from build123d import *

# Parameters (mm, degrees)
F0_W     = 31
F0_H     = 70
F0_H_2   = 17
F0_H_3   = 50
F0_H_4   = 20
F1_DEPTH = 0.4


with BuildPart() as f1:
    # F0 (on Top) → F1 (new body, symmetric)
    with BuildSketch(Plane.XY):
        Polygon((-8.5, -35), (8.5, -35), (13.5, 15), (8.5, 35), (-8.5, 35), align=None)
        with Locations((-24, 0)):
            Rectangle(F0_W, F0_H)
        with Locations((-24, -43.5)):
            Rectangle(F0_W, F0_H_2)
        Polygon((-56.5, -35), (-39.5, -35), (-39.5, 35), (-56.5, 35), (-61.5, 15), align=None)
        with Locations((-24, -77)):
            Rectangle(F0_W, F0_H_3)
        with Locations((-24, -112)):
            Rectangle(F0_W, F0_H_4)
        with Locations((-24, -130.5)):
            Rectangle(F0_W, F0_H_2)
    extrude(amount=F1_DEPTH, both=True)


solid = f1.part
Can you work these out from the model? Positions are in its coordinate system, mm. Round coordinates to 2 decimals unless told otherwise and drop trailing zeros. Loops run counter-clockwise (first coordinate to the right, second up) from the corner with the lowest first, then second, coordinate; pieces in that order, holes last. Notation, with made-up numbers: (88, -8.5) - (143, -8.5) arc R8 ccw to (143, -4.5) - close; hole circle Ø7 at (-29.5, 89.5). An arc over 180 degrees is marked (long way). Answer in a Markdown table with one row per item. Add a question column.
Q1. I want a section at A-A on z = 0.15. List the corners of the cut face in (x, y) for me.
Q2. I want a section at C-C on y = -7.5. List the corners of the cut face in (x, z) for me.
Q3. I need wall thicknesses on L1, parallel to Y at x = -46.5, z = -0.3; L2, parallel to X at y = -62.5, z = -0.05; L3, parallel to X at y = -19, z = -0.3. Which ranges of each line are inside material? Lowest first, please.
Q4. I want a section at B-B on x = -6. List the corners of the cut face in (y, z) for me.
A:
| question | item | result |
|---|---|---|
| 1 | outline | (-61.5, 15) - (-56.5, -35) - (-39.5, -35) - (-39.5, -139) - (-8.5, -139) - (-8.5, -35) - (8.5, -35) - (13.5, 15) - (8.5, 35) - (-56.5, 35) - close |
| 2 | outline | (-59.25, -0.4) - (11.25, -0.4) - (11.25, 0.4) - (-59.25, 0.4) - close |
| 3 | L1 | -35 to 35 |
| 3 | L2 | -39.5 to -8.5 |
| 3 | L3 | -58.1 to 10.1 |
| 4 | outline | (-35, -0.4) - (35, -0.4) - (35, 0.4) - (-35, 0.4) - close |
